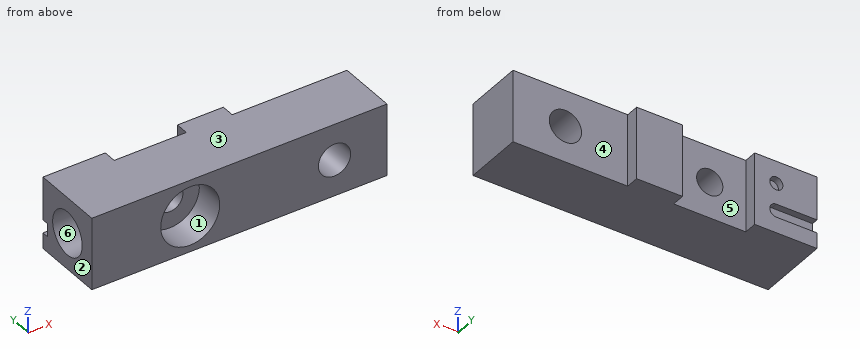
Autodesk Inventor part; units mm, degrees
ref_plane "YZ Plane" through (0, 0, 0) normal (1, 0, 0) x (0, 1, 0)
ref_plane "XZ Plane" through (0, 0, 0) normal (0, 1, 0) x (-1, 0, 0)
ref_plane "XY Plane" through (0, 0, 0) normal (0, 0, 1) x (1, 0, 0)
sketch "Boceto1" plane through (0, 0, 0) normal (0, 0, 1) x (1, 0, 0)
  line L0 (0, 0) -> (-45, 0)
  line L1 (-45, 0) -> (-45, 11)
  line L2 (0, 9) -> (0, 0)
  line L3 (-35.5, 11) -> (-35.5, 9)
  line L4 (-35.5, 9) -> (-24.5, 9)
  line L5 (-24.5, 9) -> (-24.5, 11)
  line L6 (-17.5, 11) -> (-17.5, 9)
  line L7 (-17.5, 9) -> (0, 9)
  line L8 (-45, 11) -> (-35.5, 11)
  line L9 (-24.5, 11) -> (-17.5, 11)
  dimension "d0" = 9
  dimension "d1" = 11
  dimension "d2" = 9.5
  dimension "d3" = 7
  dimension "d4" = 17.5
  dimension "d5" = 11
  dimension "d6" = 2
  dimension "d7" = 2
extrude "Extrusión1" add sketch "Boceto1" along normal blind 11
sketch "Boceto2" plane through (-45, 0, 0) normal (0, -1, 0) x (1, 0, 0)
  line L0 (0, 0) -> (45, 0)
  line L1 (45, 0) -> (45, 11)
  line L2 (0, 11) -> (45, 11)
  line L3 (0, 0) -> (0, 11)
  line L4 (45, 5.5) -> (0, 5.5) construction
  line L5 (45, 11) -> (27.5, 11)
  line L6 (37, 11) -> (37, 0) construction
  line L7 (15, 11) -> (15, 0) construction
  line L8 (0, 0) -> (45, 0)
  circle A0 centre (37, 5.5) radius 2.85
  circle A1 centre (15, 5.5) radius 4.5
  circle A2 centre (15, 5.5) radius 2
  dimension "d10" = 8
  dimension "d11" = 22
  dimension "d12" = 9
  dimension "d13" = 4
  dimension "d14" = 5.7
hole "Agujero1" at (-8, 0, 5.5) direction (0, 1, 0) diameter 4.917 end through all
hole "Agujero2" at (-30, 0, 5.5) direction (0, 1, 0) diameter 4 end through all counterbore diameter 9 counterbore depth 4.6
sketch "Boceto3" plane through (-45, 11, 0) normal (0, 1, 0) x (1, 0, 0)
  line L0 (9.5, 0) -> (0, 0)
  line L1 (0, 0) -> (0, -11)
  line L2 (9.5, -11) -> (0, -11)
  line L3 (9.5, 0) -> (9.5, -11)
  line L4 (6.2, -3.4) -> (-0.5191, -3.4) construction
  line L5 (6.2, -4.4) -> (-0.5191, -4.4)
  line L6 (-0.5191, -2.4) -> (6.2, -2.4)
  arc A0 (6.2, -4.4) -> (6.2, -2.4) centre (6.2, -3.4) ccw
  arc A1 (-0.5191, -2.4) -> (-0.5191, -4.4) centre (-0.5191, -3.4) ccw
  line L7 (9.5, -5.5) -> (0, -5.5) construction
  circle A2 centre (6.2, -7.6) radius 1
  point P0 (45, 0)
  point P1 (2.8405, -3.4)
  dimension "d29" = 2.1
  dimension "d30" = 2
  dimension "d31" = 6.2
  dimension "d32" = 2.1
  dimension "d33" = 2
  dimension "d34" = 6.2
extrude "Extrusión2" cut sketch "Boceto3" against normal blind 1 contours L6 A0 L5 L1 | L1 L5 A1 L6 | A2
sketch "Boceto4" plane through (-45, 0, 0) normal (-1, 0, 0) x (0, 0, 1)
  line L0 (4.4, 11) -> (4.4, 10)
  line L1 (4.4, 10) -> (2.4, 10)
  line L2 (2.4, 10) -> (2.4, 11)
  line L3 (0, 11) -> (2.4, 11)
  line L4 (0, 11) -> (0, 0)
  line L5 (0, 0) -> (11, 0)
  line L6 (11, 11) -> (11, 0)
  line L7 (4.4, 11) -> (11, 11)
  line L8 (11, 5.5) -> (0, 5.5) construction
  line L9 (0, 11) -> (0, 0)
  line L10 (5.5, 0) -> (5.5, 11) construction
  point P0 (5.5, 5.5)
hole "Agujero3" at (-45, 5.5, 5.5) direction (1, 0, 0) diameter 6.647 depth 8
properties part number "Hudson 1-55"
The model under review builds one solid part; all positions refer to its coordinate system, in mm. Face numbers are marked on the shaded views. A direction names the side the tool comes from. Round coordinates to 2 decimals unless told otherwise and drop trailing zeros. Loops run counter-clockwise (first coordinate to the right, second up) from the corner with the lowest first, then second, coordinate; pieces in that order, holes last. Notation, with made-up numbers: (-26, 33.5) -> (10, 33.5) arc R20 ccw to (10, 47.5) -> close; hole circle Ø8 at (65.5, 55). An arc over 180 degrees is marked (long way). Answer as CSV lines item,"result".
1) Add section C-C on y = 5.5. Write out the cut boundary in (x, z), plus the area to 3 significant figures.
Geometry results:
outline,"(-45, 0) -> (0, 0) -> (0, 11) -> (-45, 11) -> (-45, 8.82) -> (-37, 8.82) -> (-37, 2.18) -> (-45, 2.18) -> close; hole circle Ø4 at (-30, 5.5); hole circle Ø4.92 at (-8, 5.5)"
area,"410 mm²"
2) Tool access review of the marked faces 4, 5 and 6: name each direction out of +Z, -Z, +X, -X, +Y, -Y from which nothing blocks a thin tool from reaching the whole face with its end or side.
Geometry results:
face 4,"+Z, -Z, +X, +Y"
face 5,"+Z, -Z, +Y"
face 6,"-X"
3) Add section B-B on x = -30. Write out the cut boundary in (y, z), plus the area to 3 significant figures.
Geometry results:
outline,"(0, 0) -> (9, 0) -> (9, 3.5) -> (4.6, 3.5) -> (4.6, 1) -> (0, 1) -> close; (0, 10) -> (4.6, 10) -> (4.6, 7.5) -> (9, 7.5) -> (9, 11) -> (0, 11) -> close"
area,"40.0 mm²"
4) To check wall thickness, follow line 1 along X through (y, z) = (5, 5.5); line 2 along Z through (x, y) = (-8, 3.75); line 3 along X through (y, z) = (1.5, 5). State the ranges of each line that lie inside material, in increasing order. Write a range as from..to.
Geometry results:
line 1,"x = -37..-32, -28..-10.46, -5.54..0"
line 2,"z = 0..3.04, 7.96..11"
line 3,"x = -45..-34.47, -25.53..-10.41, -5.59..0"
5) Add section D-D on y = 1. Write out the cut boundary in (x, z).
Geometry results:
outline,"(-45, 0) -> (0, 0) -> (0, 11) -> (-45, 11) -> close; hole circle Ø9 at (-30, 5.5); hole circle Ø4.92 at (-8, 5.5)"
6) Add section A-A on z = 5.5. Write out the cut boundary in (x, y), plus the area to 3 significant figures.
Geometry results:
outline,"(-45, 0) -> (-34.5, 0) -> (-34.5, 4.6) -> (-32, 4.6) -> (-32, 9) -> (-35.5, 9) -> (-35.5, 11) -> (-45, 11) -> (-45, 8.82) -> (-37, 8.82) -> (-37, 2.18) -> (-45, 2.18) -> close; (-28, 4.6) -> (-25.5, 4.6) -> (-25.5, 0) -> (-10.46, 0) -> (-10.46, 9) -> (-17.5, 9) -> (-17.5, 11) -> (-24.5, 11) -> (-24.5, 9) -> (-28, 9) -> close; (-5.54, 0) -> (0, 0) -> (0, 9) -> (-5.54, 9) -> close"
area,"282 mm²"
7) Draft analysis for pull direction Z (two halves, no side actions). For the marked faces 1, 2 and 3, state which applies: pulls with the +Z half, pulls with the -Z half, needs draft (parallel to the pull), parting line crosses it, or undercut.
Geometry results:
face 1,"undercut"
face 2,"needs draft"
face 3,"pulls with the +Z half"
8) For P1, Ø5, axis at x = -37, y = 1.5, coming from the -Z side; P2, Ø1, axis at y = 6, z = 3, coming from the -X side; P3, Ø2, axis at x = -5.5, z = 9, coming from the +Y side; P4, Ø1.6, axis at x = -40.5, z = 3.5, coming from the +Y side, all flat-tipped, find the tip position at first contact; note any pin that passes through.
Geometry results:
P1,"stops at z = 0"
P2,"stops at x = -37"
P3,"stops at y = 9"
P4,"stops at y = 10"
